Here's how the part is built. I have some questions about the finished solid (model axes, mm). Round coordinates to 2 decimals unless told otherwise and drop trailing zeros. Order: outer loops, then holes, each group sorted by start corner. A loop starts at its lowest first (then second) coordinate and runs counter-clockwise, first axis right, second up.
```python
from build123d import *

# Parameters (mm, degrees)
F0_R     = 79
F1_DEPTH = 1


with BuildPart() as f1:
    # F0 (on Front) → F1 (new body)
    with BuildSketch(Plane.XZ):
        Circle(F0_R)
        with BuildLine():
            ThreePointArc((6.9882765021, 60.0950413223), (42.7799602618, 42.7799602618), (60.0950413223, 6.9882765021))
            ThreePointArc((60.0950413223, 6.9882765021), (65.3044400952, 5.0909090909), (67.5, 0))
            ThreePointArc((67.5, 0), (65.3044400952, -5.0909090909), (60.0950413223, -6.9882765021))
            ThreePointArc((60.0950413223, -6.9882765021), (42.7799602618, -42.7799602618), (6.9882765021, -60.0950413223))
            ThreePointArc((6.9882765021, -60.0950413223), (6.9970685117, -60.2974358305), (7, -60.5))
            ThreePointArc((7, -60.5), (-0.2025641695, -67.4970685117), (-6.9882765021, -60.0950413223))
            ThreePointArc((-6.9882765021, -60.0950413223), (-42.7799602618, -42.7799602618), (-60.0950413223, -6.9882765021))
            ThreePointArc((-60.0950413223, -6.9882765021), (-67.5, 0), (-60.0950413223, 6.9882765021))
            ThreePointArc((-60.0950413223, 6.9882765021), (-42.7799602618, 42.7799602618), (-6.9882765021, 60.0950413223))
            ThreePointArc((-6.9882765021, 60.0950413223), (-0.2025641695, 67.4970685117), (7, 60.5))
            ThreePointArc((7, 60.5), (6.9970685117, 60.2974358305), (6.9882765021, 60.0950413223))
        make_face(mode=Mode.SUBTRACT)
        with BuildLine():
            ThreePointArc((60.0950413223, -6.9882765021), (53.5, 0), (60.0950413223, 6.9882765021))
            ThreePointArc((60.0950413223, 6.9882765021), (42.7799602618, 42.7799602618), (6.9882765021, 60.0950413223))
            ThreePointArc((6.9882765021, 60.0950413223), (4.8044400952, 55.4090909091), (0, 53.5))
            ThreePointArc((0, 53.5), (-4.8044400952, 55.4090909091), (-6.9882765021, 60.0950413223))
            ThreePointArc((-6.9882765021, 60.0950413223), (-42.7799602618, 42.7799602618), (-60.0950413223, 6.9882765021))
            ThreePointArc((-60.0950413223, 6.9882765021), (-55.4090909091, 4.8044400952), (-53.5, 0))
            ThreePointArc((-53.5, 0), (-55.4090909091, -4.8044400952), (-60.0950413223, -6.9882765021))
            ThreePointArc((-60.0950413223, -6.9882765021), (-42.7799602618, -42.7799602618), (-6.9882765021, -60.0950413223))
            ThreePointArc((-6.9882765021, -60.0950413223), (0, -53.5), (6.9882765021, -60.0950413223))
            ThreePointArc((6.9882765021, -60.0950413223), (42.7799602618, -42.7799602618), (60.0950413223, -6.9882765021))
        make_face()
        with BuildLine():
            ThreePointArc((39.5, 0), (-27.9307178569, -27.9307178569), (0, 39.5))
            ThreePointArc((0, 39.5), (27.9307178569, 27.9307178569), (39.5, 0))
        make_face(mode=Mode.SUBTRACT)
    extrude(amount=F1_DEPTH)


solid = f1.part
```
1) If we section it at B-B (x = -28.5): Write out the boundary of the cut face in (y, z), plus the area to 3 significant figures.
2) I need wall thicknesses on line 1 (X direction, y = -0.7, z = 1.5); line 2 (X direction, y = -0.1, z = -2); line 3 (X direction, y = -0.1, z = 36). Which ranges of each line are inside material? Lowest first, please.
3) If we section it at D-D (x = -2.5): Write out the boundary of the cut face in (y, z), plus the area to 3 significant figures.
4) If we section it at C-C (z = -25): Write out the boundary of the cut face in (x, y), plus the area to 3 significant figures.
5) If we section it at A-A (y = -0.3): Write out the boundary of the cut face in (x, z), plus the area to 3 significant figures.
Solutions:
1. outline: (-1, -73.68) - (0, -73.68) - (0, -27.35) - (-1, -27.35) - close; (-1, 27.35) - (0, 27.35) - (0, 73.68) - (-1, 73.68) - close
1. area: 92.7 mm2
2. line 1: x = -78.99 to -67.34, -53.66 to -39.47, 39.47 to 53.66, 67.34 to 78.99
2. line 2: x = -78.97 to -67.21, -53.79 to -39.45, 39.45 to 53.79, 67.21 to 78.97
2. line 3: x = -70.32 to -16.26, 16.26 to 70.32
3. outline: (-1, -78.96) - (0, -78.96) - (0, -67.04) - (-1, -67.04) - close; (-1, -53.96) - (0, -53.96) - (0, -39.42) - (-1, -39.42) - close; (-1, 39.42) - (0, 39.42) - (0, 53.96) - (-1, 53.96) - close; (-1, 67.04) - (0, 67.04) - (0, 78.96) - (-1, 78.96) - close
3. area: 52.9 mm2
4. outline: (-74.94, -1) - (-30.58, -1) - (-30.58, 0) - (-74.94, 0) - close; (30.58, -1) - (74.94, -1) - (74.94, 0) - (30.58, 0) - close
4. area: 88.7 mm2
5. outline: circle Ø158 at (0, 0); hole circle Ø14 at (-60.5, 0); hole circle Ø79 at (0, 0); hole circle Ø14 at (0, -60.5); hole circle Ø14 at (0, 60.5); hole circle Ø14 at (60.5, 0)
5. area: 14,100 mm2
